Read the model definition and answer for the solid it produces. Units are mm, in the model's axes. Face numbers are marked on the shaded views. A direction names the side the tool comes from. Give positions to 0.01 mm unless a question says otherwise; leave off trailing zeros. Loops run counter-clockwise (first coordinate to the right, second up) from the corner with the lowest first, then second, coordinate; pieces in that order, holes last. Notation, with made-up numbers: M 19,0 L 57,0 A21 ccw 57,25 Z; hole C -24,50 d9. An arc over 180 degrees is marked long. Return JSON: item names as keys, results as strings. Group by question number.
```python
from build123d import *

# Parameters (mm, degrees)
SKETCH1_R           = 31
BOSS_EXTRUDE1_DEPTH = 5
SKETCH2_R           = 2
CUT_EXTRUDE1_DEPTH  = 12.5
SKETCH5_W           = 17.462022727
SKETCH5_H           = 5.971364383
CUT_EXTRUDE3_DEPTH  = 5
SKETCH6_R           = 5
CUT_EXTRUDE4_DEPTH  = 5


with BuildPart() as part:
    # Sketch1 → Boss-Extrude1 (new body)
    with BuildSketch(Plane(origin=(0, 0, 0), x_dir=(1, 0, 0), z_dir=(0, 1, 0))):
        with Locations(Location((0, 0, 0), (0, 0, 270))):
            Circle(SKETCH1_R)
    extrude(amount=BOSS_EXTRUDE1_DEPTH)

    # Sketch2 → Cut-Extrude1 (cut)
    with BuildSketch(Plane(origin=(0, 5, 0), x_dir=(1, 0, 0), z_dir=(0, 1, 0))):
        with Locations(Location((-26.719955328, -5.965376271, 0), (0, 0, 270))):
            Circle(SKETCH2_R)
        with Locations(Location((-5.965376271, 26.719955328, 0), (0, 0, 270))):
            Circle(SKETCH2_R)
        with Locations(Location((26.719955328, 5.965376271, 0), (0, 0, 270))):
            Circle(SKETCH2_R)
        with Locations(Location((5.965376271, -26.719955328, 0), (0, 0, 270))):
            Circle(SKETCH2_R)
    extrude(amount=-CUT_EXTRUDE1_DEPTH, mode=Mode.SUBTRACT)

    # Sketch5 → Cut-Extrude3 (cut)
    with BuildSketch(Plane(origin=(0, 5, 0), x_dir=(1, 0, 0), z_dir=(0, 1, 0))):
        with Locations((13.983311231, 16.066566387)):
            Rectangle(SKETCH5_W, SKETCH5_H)
    extrude(amount=-CUT_EXTRUDE3_DEPTH, mode=Mode.SUBTRACT)

    # Sketch6 → Cut-Extrude4 (cut)
    with BuildSketch(Plane(origin=(0, 5, 0), x_dir=(1, 0, 0), z_dir=(0, 1, 0))):
        with Locations(Location((-7.372449441, -14.438403546, 0), (0, 0, 270))):
            Circle(SKETCH6_R)
        with Locations(Location((14.753523974, -5.51293548, 0), (0, 0, 270))):
            Circle(SKETCH6_R)
    extrude(amount=-CUT_EXTRUDE4_DEPTH, mode=Mode.SUBTRACT)


solid = part.part
```
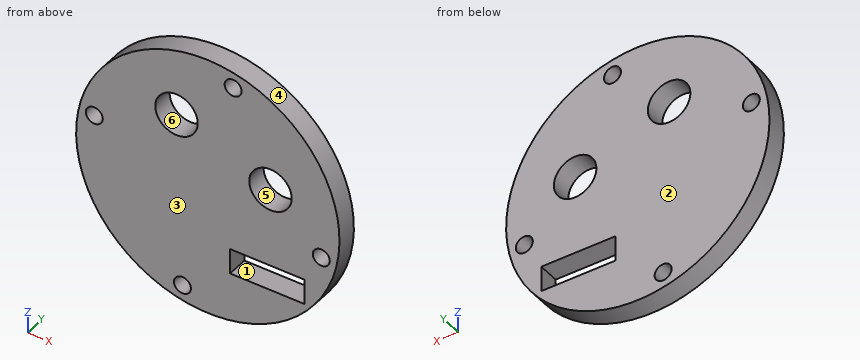
1. For the marked faces 1 and 2, determine the directions among +Z, -Z, +X, -X, +Y, -Y from which every point of the face is accessible in a straight line to the end or side of a thin tool.
2. Find section C-C (x = -25.5). Write down the section's boundary in (y, z), and give its area (3 significant figures).
3. Straight lines are drawn through the part: line 1 along X through (y, z) = (4.2, 7.5); line 2 along Z through (x, y) = (6, 1.1); line 3 along Z through (x, y) = (19, 1.4). For each, find the intervals that lie inside material, in ascending order.
4. Find section D-D (z = 27). Write down the section's boundary in (x, y), and give its area (3 significant figures).
5. Find section A-A (x = 17.5). Write down the section's boundary in (y, z), and give its area (3 significant figures).
6. The mould has two halves that part along X. Classify the marked faces 3, 4, 5 and 6: +X half, -X half, draft (parallel to the pull), parting line (faces both ways), or undercut.
7. Find section B-B (z = 7). Write down the section's boundary in (x, y), and give its area (3 significant figures).
8. Flat-ended cylindrical pins translate along their axes: P1, Ø1.5, axis at y = 2.5, z = -15.5, coming from the +X side; P2, Ø2, axis at x = 8, y = 3.5, coming from the +Z side; P3, Ø2, axis at x = -6.5, y = 3, coming from the +Z side. Find the tip coordinate at first contact, or state that the pin passes through.
Result:
{
 "1": {"face 1": "+Y, -Y", "face 2": "+Z, -Z, +X, -X, +Y"},
 "2": {"outline": "M 0,-17.63 L 5,-17.63 L 5,4.38 L 0,4.38 Z; M 0,7.55 L 5,7.55 L 5,17.63 L 0,17.63 Z", "area": "160 mm2"},
 "3": {"line 1": "x = -30.08 to -28, -25.44 to 10.17, 19.34 to 30.08", "line 2": "z = -30.41 to -19.05, -13.08 to 24.72, 28.72 to 30.41", "line 3": "z = -24.49 to -19.05, -13.08 to 2.87, 8.15 to 24.49"},
 "4": {"outline": "M -15.23,0 L 3.99,0 L 3.99,5 L -15.23,5 Z; M 7.95,0 L 15.23,0 L 15.23,5 L 7.95,5 Z", "area": "133 mm2"},
 "5": {"outline": "M 0,-25.59 L 5,-25.59 L 5,-19.05 L 0,-19.05 Z; M 0,-13.08 L 5,-13.08 L 5,1.33 L 0,1.33 Z; M 0,9.69 L 5,9.69 L 5,25.59 L 0,25.59 Z", "area": "184 mm2"},
 "6": {"face 3": "draft", "face 4": "parting line", "face 5": "undercut", "face 6": "undercut"},
 "7": {"outline": "M -30.2,0 L -28.43,0 L -28.43,5 L -30.2,5 Z; M -25.01,0 L 9.98,0 L 9.98,5 L -25.01,5 Z; M 19.53,0 L 30.2,0 L 30.2,5 L 19.53,5 Z", "area": "237 mm2"},
 "8": {"P1": "stops at x = 27.27", "P2": "stops at z = 30.2", "P3": "stops at z = 30.51"}
}
